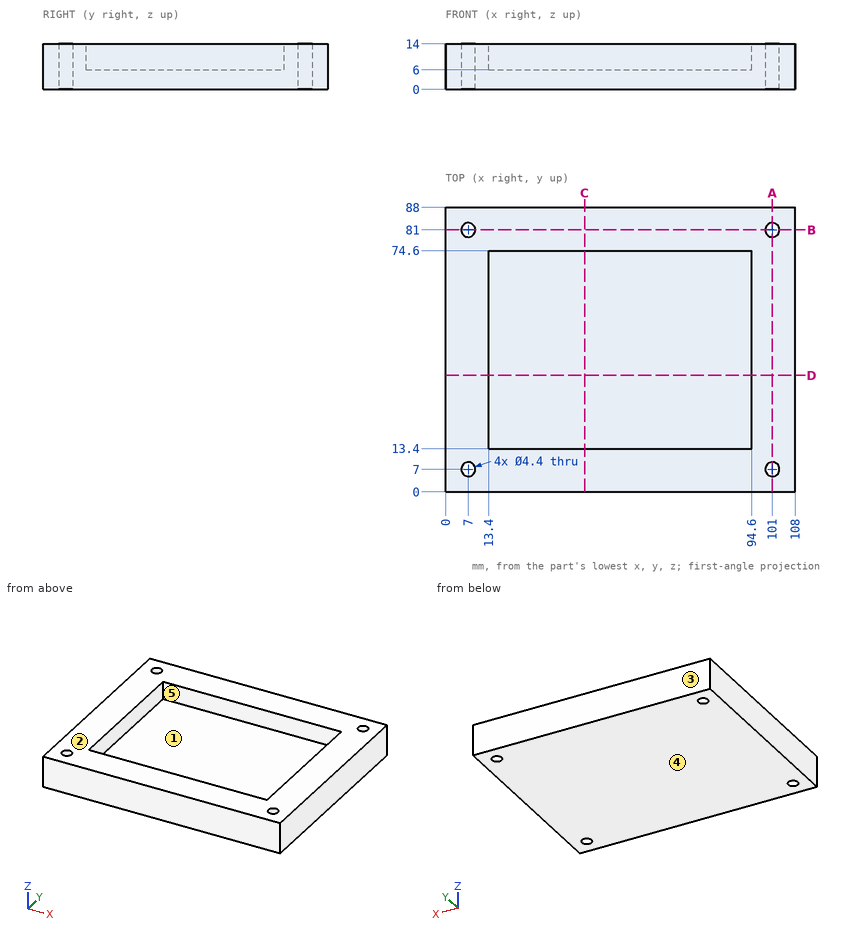
Design review of the part shown in the three views and the two pictorial views. Dimensions are in mm from the part's minimum x, y and z. A direction names the side the tool comes from. Round coordinates to 2 decimals unless told otherwise and drop trailing zeros. Write each loop counter-clockwise with the first axis right and the second up, starting at its lowest first coordinate (ties: lowest second). Pieces come first, ordered by that corner, then holes. Notation, with made-up numbers: (-4, -15.75) -> (40, -15.75) arc R26 cw to (40, 3.25) -> close; hole circle Ø9 at (-32, 10.25). An arc over 180 degrees is marked (long way). Write item = value, one per line. Start each with the question number.
1) Tool access review of the marked faces 1 and 2: name each direction out of +Z, -Z, +X, -X, +Y, -Y from which nothing blocks a thin tool from reaching the whole face with its end or side.
2) Take a section at A-A, the plane x = 101. State the section outline as (y, z) points.
3) Clearance check with flat-ended pins moving along their axes: pin 1 (8 mm diameter, centred on y = 24, z = 3.5, fed in from -X); pin 2 (6 mm diameter, centred on x = 67.5, y = 62.5, fed in from +Z). State where each tip first meets the part, or that it passes through.
4) Wall thickness on probe 1 along Y at (x, z) = (101, 3.5); probe 2 along X at (y, z) = (25, 13.25); probe 3 along X at (y, z) = (81, 4.5): over which ranges is each line inside the solid? List them lowest first. Write a range as from..to.
5) Take a section at B-B, the plane y = 81. State the section outline as (x, z) points.
6) Take a section at D-D, the plane y = 36. State the section outline as (x, z) points, plus the area to 3 significant figures.
7) Take a section at C-C, the plane x = 43. State the section outline as (y, z) points, plus the area to 3 significant figures.
8) Mouldability with a two-part tool opening along Y and no side actions: class the marked faces 3, 4 and 5 as +Y half, -Y half, draft (parallel to the pull), parting line (faces both ways), or undercut.
Results list:
q1.face_1 = +Z
q1.face_2 = +Z, +X, -X, +Y, -Y
q2.outline = (0, 0) -> (4.8, 0) -> (4.8, 14) -> (0, 14) -> close; (9.2, 0) -> (78.8, 0) -> (78.8, 14) -> (9.2, 14) -> close; (83.2, 0) -> (88, 0) -> (88, 14) -> (83.2, 14) -> close
q3.pin_1 = 0
q3.pin_2 = 6
q4.probe_1 = 0..4.8, 9.2..78.8, 83.2..88
q4.probe_2 = 0..13.4, 94.6..108
q4.probe_3 = 0..4.8, 9.2..98.8, 103.2..108
q5.outline = (0, 0) -> (4.8, 0) -> (4.8, 14) -> (0, 14) -> close; (9.2, 0) -> (98.8, 0) -> (98.8, 14) -> (9.2, 14) -> close; (103.2, 0) -> (108, 0) -> (108, 14) -> (103.2, 14) -> close
q6.outline = (0, 0) -> (108, 0) -> (108, 14) -> (94.6, 14) -> (94.6, 6) -> (13.4, 6) -> (13.4, 14) -> (0, 14) -> close
q6.area = 862 mm²
q7.outline = (0, 0) -> (88, 0) -> (88, 14) -> (74.6, 14) -> (74.6, 6) -> (13.4, 6) -> (13.4, 14) -> (0, 14) -> close
q7.area = 742 mm²
q8.face_3 = +Y half
q8.face_4 = draft
q8.face_5 = undercut
